Here's how the part is built. I have some questions about the finished solid (model axes, mm). Face numbers are marked on the shaded views. A direction names the side the tool comes from. Round coordinates to 2 decimals unless told otherwise and drop trailing zeros. Loops run counter-clockwise (first coordinate to the right, second up) from the corner with the lowest first, then second, coordinate; pieces in that order, holes last. Notation, with made-up numbers: M 24,-20.5 L 77,-20.5 A32 cw 77,11.5 Z; hole C -36,32.5 d11. An arc over 180 degrees is marked long. Use a Markdown table: item, result.
from build123d import *

# Parameters (mm, degrees)
F1_DEPTH = 25.4


with BuildPart() as f1:
    # F0 (on Right) → F1 (new body)
    with BuildSketch(Plane.YZ):
        Polygon((8.753066, -50.786357), (13.879089, -35.358516), (-43.346036, -0.368352), (-44.144051, -0.641464), (-52.029345, -13.493421), align=None)
        Polygon((-67.410849, -8.604288), (-52.029345, -13.493421), (-44.144051, -0.641464), align=None)
        Polygon((43.804381, -50.786357), (43.804381, 54.707926), (13.879089, -35.358516), (8.753066, -50.786357), align=None)
    extrude(amount=F1_DEPTH)


solid = f1.part
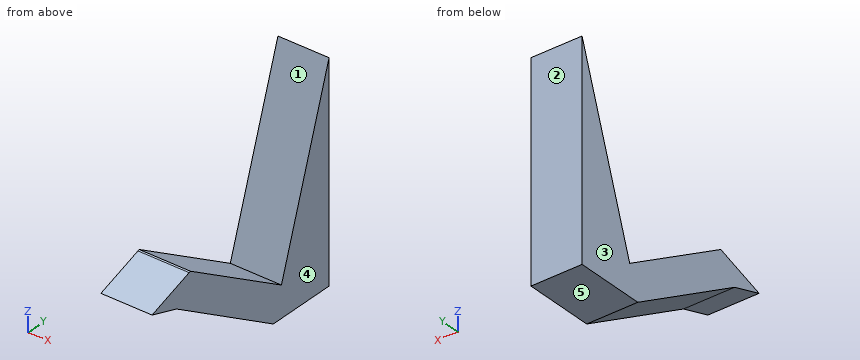
1. Imagine slicing it at C-C, the plane z = -2. Write out the boundary of the cut face in (x, y), then the cut area to 3 significant figures.
Answer sheet:
| item | result |
|---|---|
| outline | M 0,-48.11 L 25.4,-48.11 L 25.4,-40.68 L 0,-40.68 Z; M 0,24.96 L 25.4,24.96 L 25.4,43.8 L 0,43.8 Z |
| area | 667 mm2 |
2. Imagine slicing it at A-A, the plane z = -15. Write out the boundary of the cut face in (x, y).
Answer sheet:
| item | result |
|---|---|
| outline | M 0,-49.57 L 25.4,-49.57 L 25.4,-19.42 L 0,-19.42 Z; M 0,20.64 L 25.4,20.64 L 25.4,43.8 L 0,43.8 Z |
3. Which directions (+Z, -Z, +X, -X, +Y, -Y) give clear straight access to the entire face, cutting with the end or side of a thin tool? Please do the marked faces 1 and 2.
Answer sheet:
| item | result |
|---|---|
| face 1 | +Z, +X, -X |
| face 2 | +Z, -Z, +X, -X, +Y |
4. Imagine slicing it at B-B, the plane x = 2.25. Write out the boundary of the cut face in (y, z), then the cut area to 3 significant figures.
Answer sheet:
| item | result |
|---|---|
| outline | M -67.41,-8.6 L -52.03,-13.49 L 8.75,-50.79 L 43.8,-50.79 L 43.8,54.71 L 13.88,-35.36 L -43.35,-0.37 L -44.14,-0.64 Z |
| area | 3,060 mm2 |
5. For pin 1 Ø4 at (x, z) = (13.5, -22.5) entering from -Y; pin 2 Ø1 at (x, z) = (16, -33.5) entering from -Y; pin 3 Ø8 at (x, y) = (21.5, -45) entering from +Z, each with a flat end and sliding along its axis, tell me the tip position at first contact or that it passes through.
Answer sheet:
| item | result |
|---|---|
| pin 1 | y = -40.61 |
| pin 2 | y = -20.24 |
| pin 3 | z = -0.37 |
6. Imagine slicing it at D-D, the plane y = -46. Write out the boundary of the cut face in (x, z).
Answer sheet:
| item | result |
|---|---|
| outline | M 0,-17.19 L 25.4,-17.19 L 25.4,-1.28 L 0,-1.28 Z |
7. I need wall thicknesses on probe 1 along Y at (x, z) = (9, -34.5); probe 2 along Y at (x, z) = (16.25, -14.5); probe 3 along Z at (x, y) = (8.25, 8.5). Which ranges of each line are inside material? Lowest first, please. Write a range as from..to.
Answer sheet:
| item | result |
|---|---|
| probe 1 | -17.79..12.48, 14.16..43.8 |
| probe 2 | -50.39..-20.23, 20.81..43.8 |
| probe 3 | -50.63..-32.07 |
8. We'd pull the mould along X, two halves only. Please class the marked faces 3, 4 and 5: +X half, -X half, draft (parallel to the pull), parting line (faces both ways), or undercut.
Answer sheet:
| item | result |
|---|---|
| face 3 | -X half |
| face 4 | +X half |
| face 5 | draft |
